from build123d import *

# Parameters (mm, degrees)
HOLE_WIZARD_6_0_6_1_D     = 6
HOLE_WIZARD_6_0_6_1_DEPTH = 6
SKETCH_4_W                = 0.75
SKETCH_4_H                = 5
FILLET_1_R                = 0.5
FILLET_2_R                = 0.7


with BuildPart() as part:
    # 草图1 → 旋转1 (revolve)
    with BuildSketch(Plane.XZ, mode=Mode.PRIVATE) as revolve_1_sk:
        Polygon((7, 1.3), (0, 1.3), (0, -11), (6, -11), (6, -2.6), (5.75, -2.6), (5.75, -2.5), (6, -2.5), (6, -2.4), (5.75, -2.4), (5.75, -2.3), (6, -2.3), (6, -2.2), (5.75, -2.2), (5.75, -2.1), (6, -2.1), (6, -2), (5.75, -2), (5.75, -1.9), (6, -1.9), (6, -1.8), (5.75, -1.8), (5.75, -1.7), (6, -1.7), (6, -1.6), (5.75, -1.6), (5.75, -1.5), (6, -1.5), (6, -1.4), (5.75, -1.4), (5.75, -1.3), (6, -1.3), (6, -1.2), (5.75, -1.2), (5.75, -1.1), (6, -1.1), (6, -1), (5.75, -1), (5.75, -0.9), (6, -0.9), (6, -0.8), (5.75, -0.8), (5.75, -0.7), (6, -0.7), (6, 0), (7, 0), align=None)
    revolve(revolve_1_sk.sketch.rotate(Axis((0, 0, 1.3), (0, 0, -1)), 180), axis=Axis((0, 0, 1.3), (0, 0, -1)))

    # Ø6.0 (6) 直径孔1
    with Locations(Plane.XY.offset(1.3)):
        with Locations((0, -2.5)):
            Hole(HOLE_WIZARD_6_0_6_1_D / 2, depth=HOLE_WIZARD_6_0_6_1_DEPTH)

    # 草图4 → 旋转2 (revolve)
    with BuildSketch(Plane(origin=(0, -2.5, 0), x_dir=(1, 0, 0), z_dir=(0, 1, 0))):
        with Locations((0.375, 2.2)):
            Rectangle(SKETCH_4_W, SKETCH_4_H)
    revolve(axis=Axis((0, -2.5, -4.7), (0, 0, 1)))

    # 圆角1
    fillet_1_edges = [part.edges().sort_by_distance(p)[0] for p in [
        (7, 0, 0),
        (6, 0, -11),
        (7, 0, 1.3),
    ]]
    fillet(fillet_1_edges, radius=FILLET_1_R)

    # 圆角2
    fillet_2_edges = [part.edges().sort_by_distance(p)[0] for p in [
        (-0.75, -2.5, 0.3),
    ]]
    fillet(fillet_2_edges, radius=FILLET_2_R)


solid = part.part
CAD build for the part. Positions are in the model's coordinates, mm. A direction names the side the tool comes from. Round coordinates to 2 decimals unless told otherwise and drop trailing zeros. Write each loop counter-clockwise with the first axis right and the second up, starting at its lowest first coordinate (ties: lowest second). Pieces come first, ordered by that corner, then holes.
(1) Probe line 1 along Y through (x, z) = (0, -3.5); line 2 along Y through (x, z) = (0, -2.55); line 3 along Z through (x, y) = (-0.75, -0.75). List the from-to ranges inside material, lowest first.
(2) Slice it at A-A, the plane z = -4. Write the cut outline in (x, y).
(3) 3-axis set-ups, long thin cutter, end or side, ignore diameter. For faces 1 (the face through (-3.23, -6.21, 0.65)), 2 (the face through (-5.723, 1.802, -0.345)): which of +Z, -Z, +X, -X, +Y, -Y reach the whole face in a straight line?
(4) Slice it at B-B, the plane z = -8.25. Write the cut outline in (x, y).
(5) Drop flat-ended pins along their axis: P1, Ø6, axis at x = -5, y = -5, coming from the +Z side; P2, Ø1.5, axis at y = -1, z = -1.5, coming from the +X side. Give the stop position or say it passes through.
From the geometry:
1. line 1: y = -6 to -5.5, -3.25 to -1.75, 0.5 to 6
1. line 2: y = -5.75 to -5.5, -3.25 to -1.75, 0.5 to 5.75
1. line 3: z = -11 to -4.7
2. outline: circle Ø12 at (0, 0); circle Ø1.5 at (0, -2.5); hole circle Ø6 at (0, -2.5)
3. face 1: +Z, -Z
3. face 2: -Z
4. outline: circle Ø12 at (0, 0)
5. P1: stops at z = 1.3
5. P2: stops at x = 5.99
